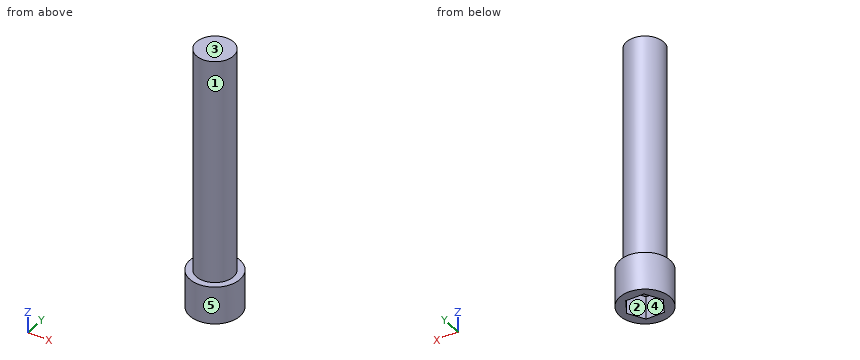
from build123d import *

# Parameters (mm, degrees)
SKETCH1_R      = 2
EXTRUDE1_DEPTH = 3
EXTRUDE3_DEPTH = 1.82
SKETCH2_R      = 1.475
EXTRUDE2_DEPTH = 18


with BuildPart() as part:
    # Sketch1 → Extrude1 (new body)
    with BuildSketch(Plane.XY):
        Circle(SKETCH1_R)
    extrude(amount=EXTRUDE1_DEPTH)

    # Sketch3 → Extrude3 (cut)
    with BuildSketch(Plane(origin=(0, 0, 0), x_dir=(-1, 0, 0), z_dir=(0, 0, -1))):
        Polygon((-1.443375673, 0), (-0.721687836, -1.25), (0.721687836, -1.25), (1.443375673, 0), (0.721687836, 1.25), (-0.721687836, 1.25), align=None)
    extrude(amount=-EXTRUDE3_DEPTH, mode=Mode.SUBTRACT)

    # Sketch2 → Extrude2 (add)
    with BuildSketch(Plane.XY.offset(3)):
        Circle(SKETCH2_R)
    extrude(amount=EXTRUDE2_DEPTH)


solid = part.part
The model under review builds one solid part; all positions refer to its coordinate system, in mm. Face numbers are marked on the shaded views. A direction names the side the tool comes from. Give positions to 0.01 mm unless a question says otherwise; leave off trailing zeros. Order: outer loops, then holes, each group sorted by start corner. A loop starts at its lowest first (then second) coordinate and runs counter-clockwise, first axis right, second up. Notation, with made-up numbers: M -32,-31.75 L -25,-31.75 A16 cw -25,-20.75 Z; hole C -16,78 d4. An arc over 180 degrees is marked long. Answer in a Markdown table with one row per item. Add a question column.
1. Mouldability with a two-part tool opening along Y and no side actions: class the marked faces 1, 2 and 3 as released by +Y, released by -Y, zero draft, split by the parting line, or undercut.
2. Machinability: for the marked faces 4 and 5, which of the approach directions +Z, -Z, +X, -X, +Y, -Y give a long, thin tool a straight path to every point of the face, cutting with its end or side? Answer none if there is none.
3. Add section A-A on x = 0. State the section outline as (y, z) points (3 decimals).
4. To check wall thickness, follow line 1 along Z through (x, y) = (-0.8, 0.05); line 2 along Z through (x, y) = (-0.05, -1.75); line 3 along X through (y, z) = (0.85, 1.75). State the ranges of each line that lie inside material, in increasing order.
5. Add section C-C on z = 3.5. State the section outline as (x, y) points (3 decimals).
6. For pin 1 Ø2 at (x, z) = (0, 8.5) entering from -Y (3 decimals); pin 2 Ø1 at (x, z) = (-1, 13) entering from +Y; pin 3 Ø2 at (x, y) = (0.5, 0) entering from -Z; pin 4 Ø1 at (y, z) = (-1.5, 8.5) entering from +X, all flat-tipped, find the tip position at first contact; note any pin that passes through.
7. Add section B-B on y = 0.3. State the section outline as (x, z) points, plus the area to 3 significant figures.
The answers:
| question | item | result |
|---|---|---|
| 1 | face 1 | split by the parting line |
| 1 | face 2 | undercut |
| 1 | face 3 | zero draft |
| 2 | face 4 | -Z |
| 2 | face 5 | +Z, -Z |
| 3 | outline | M -2,0 L -1.25,0 L -1.25,1.82 L 1.25,1.82 L 1.25,0 L 2,0 L 2,3 L 1.475,3 L 1.475,21 L -1.475,21 L -1.475,3 L -2,3 Z |
| 4 | line 1 | 1.82 to 21 |
| 4 | line 2 | 0 to 3 |
| 4 | line 3 | -1.81 to -0.95, 0.95 to 1.81 |
| 5 | outline | C 0,0 d2.95 |
| 6 | pin 1 | y = -1.475 |
| 6 | pin 2 | y = 1.39 |
| 6 | pin 3 | z = 0 |
| 6 | pin 4 | x = 1.08 |
| 7 | outline | M -1.98,0 L -1.27,0 L -1.27,1.82 L 1.27,1.82 L 1.27,0 L 1.98,0 L 1.98,3 L 1.44,3 L 1.44,21 L -1.44,21 L -1.44,3 L -1.98,3 Z |
| 7 | area | 59.2 mm2 |
